Source: CAD feature listing. Evaluate the final solid. Frame: model axes, mm. A direction names the side the tool comes from. Give positions to 0.01 mm unless a question says otherwise; leave off trailing zeros. Order: outer loops, then holes, each group sorted by start corner. A loop starts at its lowest first (then second) coordinate and runs counter-clockwise, first axis right, second up.
from build123d import *

# Parameters (mm, degrees)
SKETCH3_R              = 9
BOSS_EXTRUDE3_DEPTH    = 25.4
CUT_EXTRUDE2_START     = -26
CUT_EXTRUDE2_OUTLINE_W = 15
CUT_EXTRUDE2_OUTLINE_H = 17.4
CUT_EXTRUDE2_DEPTH     = 26
SKETCH5_W              = 5
SKETCH5_H              = 27.5
BOSS_EXTRUDE4_DEPTH    = 10
SKETCH6_W              = 60
SKETCH6_H              = 12.5
CUT_EXTRUDE3_DEPTH     = 16
SKETCH7_W              = 25
SKETCH7_H              = 6.5
BOSS_EXTRUDE5_DEPTH    = 4
CUT_EXTRUDE4_DEPTH     = 57.081726079
SKETCH9_R              = 11
CUT_EXTRUDE5_DEPTH     = 7
CUT_EXTRUDE6_START     = -16
SKETCH5_3_R            = 0.9
CUT_EXTRUDE6_DEPTH     = 16


# Read off the part's stored shape, not the designer's step: Cut-Extrude2
with BuildPart() as part:
    # Sketch3 → Boss-Extrude3 (new body)
    with BuildSketch(Plane.XY):
        Polygon((-30, -25), (30, -25), (15, 15), (-15, 15), align=None)
        Circle(SKETCH3_R, mode=Mode.SUBTRACT)
    extrude(amount=BOSS_EXTRUDE3_DEPTH)

    # Cut-Extrude2 outline → Cut-Extrude2 (cut)
    with BuildSketch(Plane(origin=(0, 15, 0), x_dir=(1, 0, 0), z_dir=(0, 1, 0)).offset(CUT_EXTRUDE2_START)):
        with Locations((22.5, -12.7)):
            Rectangle(CUT_EXTRUDE2_OUTLINE_W, CUT_EXTRUDE2_OUTLINE_H)
        with Locations((-22.5, -12.7)):
            Rectangle(CUT_EXTRUDE2_OUTLINE_W, CUT_EXTRUDE2_OUTLINE_H)
    extrude(amount=CUT_EXTRUDE2_DEPTH, mode=Mode.SUBTRACT)

    # Sketch5 → Boss-Extrude4 (add)
    with BuildSketch(Plane(origin=(0, 0, 0), x_dir=(-1, 0, 0), z_dir=(0, 0, -1))):
        with Locations((-9.525, -11.25)):
            Rectangle(SKETCH5_W, SKETCH5_H)
        with Locations((9.525, -11.25)):
            Rectangle(SKETCH5_W, SKETCH5_H)
    extrude(amount=-BOSS_EXTRUDE4_DEPTH)

    # Sketch6 → Cut-Extrude3 (cut)
    with BuildSketch(Plane(origin=(0, 0, 0), x_dir=(-1, 0, 0), z_dir=(0, 0, -1))):
        with Locations((0, 8.75)):
            Rectangle(SKETCH6_W, SKETCH6_H)
    extrude(amount=-CUT_EXTRUDE3_DEPTH, mode=Mode.SUBTRACT)

    # Sketch7 → Boss-Extrude5 (add)
    with BuildSketch(Plane.XZ.offset(25)):
        with Locations((0, 12.7)):
            Rectangle(SKETCH7_W, SKETCH7_H)
    extrude(amount=BOSS_EXTRUDE5_DEPTH)

    # Sketch8 → Cut-Extrude4 (cut, through all)
    with BuildSketch(Plane.XZ.offset(25)):
        with BuildLine():
            Line((37.5, 9.45), (22.5, 9.45))
            ThreePointArc((22.5, 9.45), (19.25, 12.7), (22.5, 15.95))
            Line((22.5, 15.95), (37.5, 15.95))
            ThreePointArc((37.5, 15.95), (40.75, 12.7), (37.5, 9.45))
        make_face()
        with BuildLine():
            Line((-37.5, 15.95), (-22.5, 15.95))
            ThreePointArc((-22.5, 15.95), (-19.25, 12.7), (-22.5, 9.45))
            Line((-22.5, 9.45), (-37.5, 9.45))
            ThreePointArc((-37.5, 9.45), (-40.75, 12.7), (-37.5, 15.95))
        make_face()
    extrude(amount=-CUT_EXTRUDE4_DEPTH, mode=Mode.SUBTRACT)

    # Sketch9 → Cut-Extrude5 (cut)
    with BuildSketch(Plane.XY.offset(25.4)):
        Circle(SKETCH9_R)
    extrude(amount=-CUT_EXTRUDE5_DEPTH, mode=Mode.SUBTRACT)

    # Sketch5<3> → Cut-Extrude6 (cut)
    with BuildSketch(Plane(origin=(0, 0, 0), x_dir=(-1, 0, 0), z_dir=(0, 0, -1)).offset(CUT_EXTRUDE6_START)):
        with Locations((9.525, 0)):
            Circle(SKETCH5_3_R)
        with Locations((-9.525, 0)):
            Circle(SKETCH5_3_R)
    extrude(amount=CUT_EXTRUDE6_DEPTH, mode=Mode.SUBTRACT)


solid = part.part
1) Reachability of faces 1 (the face through (10.424, 0.04, 8.112)), 2 (the face through (15, -1, 15)), 3 (the face through (25, -20, 15.95)), 4 (the face through (-12, 2.5, 6)), 5 (the face through (-19, -4, 4)) from +Z, -Z, +X, -X, +Y, -Y: full face, straight path, thin tool, end or side. Return the list, or none.
Checks:
face 1: -Z
face 2: +X, +Y
face 3: +X, +Y, -Y
face 4: -Z, +X, -X, +Y
face 5: -X, +Y
2) Ray query, L1, parallel to X at y = 0, z = 9 (3 decimals); L2, parallel to X at y = -2.5, z = 9.25 (3 decimals); L3, parallel to Y at x = 0, z = 24. Return the intervals inside material, ascending.
Checks:
L1: x = -15 to -10.425, -8.625 to -7.025, 7.025 to 8.625, 10.425 to 15
L2: x = -15 to -7.025, 7.025 to 15
L3: y = -25 to -11, 11 to 15
3) Section query D-D on z = 2.5. Output: boundary loops of the cut face in (x, y) (1 decimal).
Checks:
outline: (-30, -25) - (30, -25) - (19.7, 2.5) - (7, 2.5) - (7, -5.6) arc R9 cw to (-7, -5.6) - (-7, 2.5) - (-19.7, 2.5) - close; hole circle Ø1.8 at (-9.5, 0); hole circle Ø1.8 at (9.5, 0)
4) First-contact query: pin 1 Ø5 at (x, z) = (15, 9) entering from +Y; pin 2 Ø6.5 at (y, z) = (0, 7) entering from +X; pin 3 Ø3 at (y, z) = (-18.5, 16.5) entering from -X (3 decimals); pin 4 Ø3 at (x, y) = (-18, 1.5) entering from -Z. Flat tips, straight axial feed; report the tip coordinate or a pass-through.
Checks:
pin 1: stops at y = 2.5
pin 2: stops at x = 21.09
pin 3: stops at x = -28.125
pin 4: stops at z = 0
5) Section query C-C on y = -17. Output: boundary loops of the cut face in (x, z), and give its area (3 significant figures).
Checks:
outline: (-27, 0) - (27, 0) - (27, 9.45) - (22.5, 9.45) arc R3.25 cw to (22.5, 15.95) - (27, 15.95) - (27, 25.4) - (-27, 25.4) - (-27, 15.95) - (-22.5, 15.95) arc R3.25 cw to (-22.5, 9.45) - (-27, 9.45) - close
area: 1,280 mm2
6) Pull-direction query (Z, two-part tool) for faces 6 (the face through (0, -27, 15.95)), 7 (the face through (26.062, -14.498, 3.609)), 8 (the face through (19.25, -18.1, 12.63)); classes: +Z half, -Z half, draft (parallel to the pull), parting line (faces both ways), or undercut.
Checks:
face 6: +Z half
face 7: draft
face 8: undercut
7) Section query B-B on x = 0. Output: boundary loops of the cut face in (y, z).
Checks:
outline: (-29, 9.45) - (-25, 9.45) - (-25, 0) - (-9, 0) - (-9, 18.4) - (-11, 18.4) - (-11, 25.4) - (-25, 25.4) - (-25, 15.95) - (-29, 15.95) - close; (9, 16) - (15, 16) - (15, 25.4) - (11, 25.4) - (11, 18.4) - (9, 18.4) - close
8) Section query A-A on z = 19.75. Output: boundary loops of the cut face in (x, y).
Checks:
outline: (-30, -25) - (30, -25) - (24.75, -11) - (15, -11) - (15, 15) - (-15, 15) - (-15, -11) - (-24.75, -11) - close; hole circle Ø22 at (0, 0)
